Check sheet for the modelled part. Datum: model origin and axes. Units: mm. Round coordinates to 2 decimals unless told otherwise and drop trailing zeros. Order: outer loops, then holes, each group sorted by start corner. A loop starts at its lowest first (then second) coordinate and runs counter-clockwise, first axis right, second up. Notation, with made-up numbers: (43, 65) -> (88, 65) arc R14 ccw to (88, 79) -> close; hole circle Ø8 at (17.5, 19.25). An arc over 180 degrees is marked (long way). Answer in a Markdown table with one row per item. Add a question column.
1. Sectioned sample at A-A, the plane y = 0. Record the boundary of the cut face in (x, z), then the cut area to 3 significant figures.
2. Sectioned sample at B-B, the plane z = 4.1. Record the boundary of the cut face in (x, y).
3. Sectioned sample at C-C, the plane y = -24.5. Record the boundary of the cut face in (x, z), then the cut area to 3 significant figures.
4. Material ranges on L1, parallel to Y at x = 0.25, z = 3.1; L2, parallel to Y at x = 9, z = 0.65; L3, parallel to X at y = -1.5, z = 0.3, recorded low to high. Write a range as from..to.
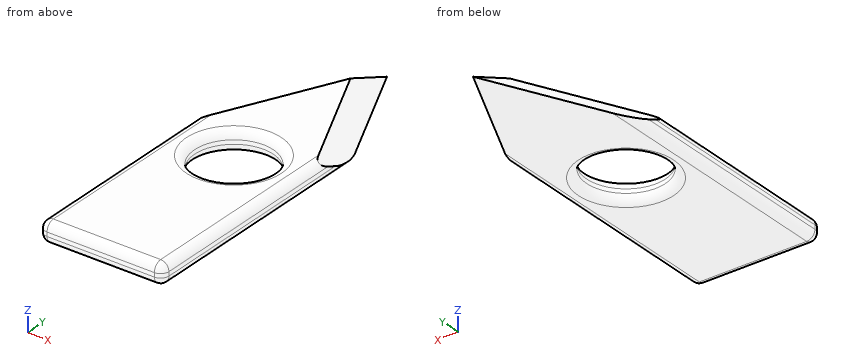
```python
from build123d import *

# Parameters (mm, degrees)
F0_W     = 30
F0_H     = 60
F0_R     = 9.5
F1_DEPTH = 5
F2_SIZE  = 4.99999
F3_R     = 2
F4_R     = 2


# Not quite as in the source:
# - a fillet or chamfer is up to 0.001 mm smaller than in the source, because OpenCascade refuses the exact size


with BuildPart() as f1:
    # F0 (on Top) → F1 (new body)
    with BuildSketch(Plane.XY):
        with Locations((0, -12.6652074978)):
            Rectangle(F0_W, F0_H)
        Circle(F0_R, mode=Mode.SUBTRACT)
        Polygon((-15, 17.3347925022), (15, 17.3347925022), (0, 49.0306541324), align=None)
    extrude(amount=F1_DEPTH)

    # F2 (size 5 in the source; OpenCascade refuses exactly that, so slightly less here)
    f2_edges = [f1.edges().sort_by_distance(p)[0] for p in [
        (-7.5, 33.182723, 5),
        (7.5, 33.182723, 5),
    ]]
    chamfer(f2_edges, length=F2_SIZE)

    # F3
    f3_edges = [f1.edges().sort_by_distance(p)[0] for p in [
        (-15, -18.509537, 5),
        (15, -18.509537, 5),
        (15, -12.665207, 0),
        (-15, -12.665207, 0),
        (-9.5, 0, 5),
        (-9.5, 0, 0),
    ]]
    fillet(f3_edges, radius=F3_R)

    # F4
    f4_edges = [f1.edges().sort_by_distance(p)[0] for p in [
        (0, -42.665207, 5),
    ]]
    fillet(f4_edges, radius=F4_R)


solid = f1.part
```
Answer key:
| question | item | result |
|---|---|---|
| 1 | outline | (-15, 2) arc R2 ccw to (-13, 0) -> (-11.5, 0) arc R2 ccw to (-9.5, 2) -> (-9.5, 3) arc R2 ccw to (-11.5, 5) -> (-13, 5) arc R2 ccw to (-15, 3) -> close; (9.5, 2) arc R2 ccw to (11.5, 0) -> (13, 0) arc R2 ccw to (15, 2) -> (15, 3) arc R2 ccw to (13, 5) -> (11.5, 5) arc R2 ccw to (9.5, 3) -> close |
| 1 | area | 48.1 mm² |
| 2 | outline | (-14.67, -40.67) arc R1.67 ccw to (-13, -42.34) -> (13, -42.34) arc R1.67 ccw to (14.67, -40.67) -> (14.67, 8.45) -> (0, 39.45) -> (-14.67, 8.45) -> close; hole circle Ø19.66 at (0, 0) |
| 3 | outline | (-15, 2) arc R2 ccw to (-13, 0) -> (13, 0) arc R2 ccw to (15, 2) -> (15, 3) arc R2 ccw to (13, 5) -> (-13, 5) arc R2 ccw to (-15, 3) -> close |
| 3 | area | 147 mm² |
| 4 | L1 | y = -42.66..-9.5, 9.5..41.26 |
| 4 | L2 | y = -42.14..-4.41, 4.41..28.49 |
| 4 | L3 | x = -14.05..-10.34, 10.34..14.05 |
